The model under review builds one solid part; all positions refer to its coordinate system, in mm. A direction names the side the tool comes from. Coordinates: 2 decimals unless noted, no trailing zeros. Order: outer loops, then holes, each group sorted by start corner. A loop starts at its lowest first (then second) coordinate and runs counter-clockwise, first axis right, second up. Notation, with made-up numbers: M 20.25,23.5 L 68.25,23.5 A22 cw 68.25,36.5 Z; hole C 62.5,22 d7. An arc over 180 degrees is marked long. Answer in a Markdown table with one row per item.
from build123d import *

# Parameters (mm, degrees)
SKETCH2_W                    = 120
SKETCH2_H                    = 8
BOSS_EXTRUDE1_DEPTH          = 12
LPATTERN1_COUNT              = 5
LPATTERN1_PITCH              = 24.25
SKETCH4_R                    = 2.05
CUT_EXTRUDE1_DEPTH           = 5
CUT_EXTRUDE1_DRAFT           = -1
CUT_EXTRUDE1_PROFILE_2_DEPTH = 5
CUT_EXTRUDE1_PROFILE_2_DRAFT = -1


with BuildPart() as part:
    # Sketch2 → Boss-Extrude1 (new body)
    with BuildSketch(Plane.XY):
        with Locations((60, 4)):
            Rectangle(SKETCH2_W, SKETCH2_H)
    extrude(amount=-BOSS_EXTRUDE1_DEPTH)

    # Sketch3 → Cut-Revolve1 (revolve, cut)
    with BuildSketch(Plane.XY):
        Polygon((8.5, 3), (9.4, 3), (9.4, 5), (2, 5), (2, 6), (11.5, 6), (11.5, 0), (9.4, 0), align=None)
    cut_revolve1 = revolve(axis=Axis((11.5, 6, 0), (0, -1, 0)), mode=Mode.SUBTRACT)

    # LPattern1: Cut-Revolve1 ×5
    with Locations(*[(i * LPATTERN1_PITCH, 0, 0) for i in range(1, LPATTERN1_COUNT)]):
        add(cut_revolve1, mode=Mode.SUBTRACT)


with BuildPart() as cut_extrude1_tool:
    # Sketch4 → Cut-Extrude1 (with draft: the straight prism first)
    with BuildSketch(Plane.XY):
        with Locations((23.5, 3)):
            Circle(SKETCH4_R)
    extrude(amount=-CUT_EXTRUDE1_DEPTH)
    # Cut-Extrude1: the draft: its side faces are tilted about the plane it starts from
    cut_extrude1_sides = [cut_extrude1_tool.faces().sort_by_distance(p)[0] for p in [
        (21.45, 3, -2.5),
    ]]
    draft(cut_extrude1_sides, Plane.XY, CUT_EXTRUDE1_DRAFT)


with BuildPart() as part_1:
    add(part.part)

    # Cut-Extrude1: cut by cut_extrude1_tool
    add(cut_extrude1_tool.part, mode=Mode.SUBTRACT)


with BuildPart() as cut_extrude1_profile_2_tool:
    # Sketch4 → Cut-Extrude1 profile 2 (with draft: the straight prism first)
    with BuildSketch(Plane.XY):
        with Locations((96.5, 3)):
            Circle(SKETCH4_R)
    extrude(amount=-CUT_EXTRUDE1_PROFILE_2_DEPTH)
    # Cut-Extrude1 profile 2: the draft: its side faces are tilted about the plane it starts from
    cut_extrude1_profile_2_sides = [cut_extrude1_profile_2_tool.faces().sort_by_distance(p)[0] for p in [
        (94.45, 3, -2.5),
    ]]
    draft(cut_extrude1_profile_2_sides, Plane.XY, CUT_EXTRUDE1_PROFILE_2_DRAFT)


with BuildPart() as part_2:
    add(part_1.part)

    # Cut-Extrude1 profile 2: cut by cut_extrude1_profile_2_tool
    add(cut_extrude1_profile_2_tool.part, mode=Mode.SUBTRACT)


solid = part_2.part
(1) Take a section at A-A (z = -7.25). Write out the cut boundary in (x, y).
Report:
| item | result |
|---|---|
| outline | M 0,0 L 120,0 L 120,8 L 0,8 Z; hole M 5.36,5 L 17.64,5 L 17.64,6 L 5.36,6 Z; hole M 29.61,5 L 41.89,5 L 41.89,6 L 29.61,6 Z; hole M 53.86,5 L 66.14,5 L 66.14,6 L 53.86,6 Z; hole M 78.11,5 L 90.39,5 L 90.39,6 L 78.11,6 Z; hole M 102.36,5 L 114.64,5 L 114.64,6 L 102.36,6 Z |
(2) Take a section at B-B (x = 108.5). Write out the cut boundary in (y, z), then the cut area to 4 significant figures.
Report:
| item | result |
|---|---|
| outline | M 0,-12 L 8,-12 L 8,0 L 6,0 L 6,-9.5 L 5,-9.5 L 5,-2.1 L 3,-2.1 L 3,-3 L 0,-2.1 Z |
| area | 74.65 mm^2 |
(3) Machinability: for faces 1 (the flat face through (23, 3, -5)), 2 (the cylindrical face through (35.7, 4, -2.1)), which of the approach directions +Z, -Z, +X, -X, +Y, -Y give a long, thin tool a straight path to every point of the face, cutting with its end or side? Answer none if there is none.
Report:
| item | result |
|---|---|
| face 1 | +Z |
| face 2 | +Z, -Y |
(4) Insertion check: P1, Ø0.9, axis at x = 36, z = -1.5, coming from the -Y side; P2, Ø2, axis at x = 97, y = 3.5, coming from the +Z side. Each pin has a flat end and moves straight along its axis. Give the tip position at first contact, or say it passes through.
Report:
| item | result |
|---|---|
| P1 | y = 6 |
| P2 | z = -5 |
(5) Take a section at C-C (x = 19). Write out the cut boundary in (y, z).
Report:
| item | result |
|---|---|
| outline | M 0,-12 L 8,-12 L 8,0 L 6,0 L 6,-5.83 L 5,-5.83 L 5,0 L 0,0 Z |
(6) To check wall thickness, follow line 1 (Y direction, x = 64.5, z = -4.5); line 2 (X direction, y = 4, z = -3.25); line 3 (Y direction, x = 108, z = -1). State the ranges of each line that lie inside material, in increasing order. Write a range as [from, to].
Report:
| item | result |
|---|---|
| line 1 | [0, 5], [6, 8] |
| line 2 | [0, 21.78], [25.22, 94.78], [98.22, 120] |
| line 3 | [6, 8] |
